Here's how the part is built. I have some questions about the finished solid (model axes, mm). Face numbers are marked on the shaded views. A direction names the side the tool comes from. Round coordinates to 2 decimals unless told otherwise and drop trailing zeros. Loops run counter-clockwise (first coordinate to the right, second up) from the corner with the lowest first, then second, coordinate; pieces in that order, holes last. Notation, with made-up numbers: M 16,84 L 34,84 A20 ccw 34,101 Z; hole C 17.5,-38 d1. An arc over 180 degrees is marked long. Write each question's results on one line, items separated by ' | '. Start each with the question number.
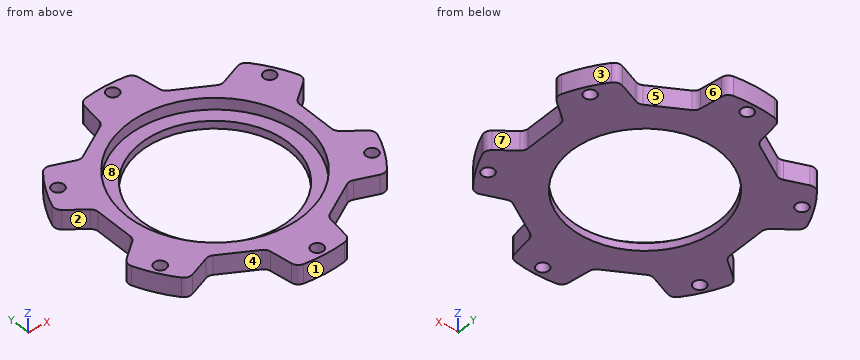
```python
from build123d import *

# Parameters (mm, degrees)
SKETCH_1_R          = 34
SKETCH_1_R_2        = 19
EXTRUDE_1_DEPTH     = 5
SKETCH_2_R          = 22.5
CUT_EXTRUDE_1_DEPTH = 3
SKETCH_3_R          = 1.55
CUT_EXTRUDE_2_DEPTH = 13
CUT_EXTRUDE_3_DEPTH = 13
FILLET_1_R          = 2


with BuildPart() as part:
    # 草图1 → 凸台-拉伸1 (new body)
    with BuildSketch(Plane.XY):
        Circle(SKETCH_1_R)
        Circle(SKETCH_1_R_2, mode=Mode.SUBTRACT)
    extrude(amount=EXTRUDE_1_DEPTH)

    # 草图2 → 切除-拉伸1 (cut)
    with BuildSketch(Plane.XY.offset(5)):
        Circle(SKETCH_2_R)
    extrude(amount=-CUT_EXTRUDE_1_DEPTH, mode=Mode.SUBTRACT)

    # 草图3 → 切除-拉伸2 (cut)
    with BuildSketch(Plane(origin=(0, 0, 0), x_dir=(-1, 0, 0), z_dir=(0, 0, -1))):
        with Locations((0, 31.5)):
            Circle(SKETCH_3_R)
        with Locations((27.279800219, 15.75)):
            Circle(SKETCH_3_R)
        with Locations((27.279800219, -15.75)):
            Circle(SKETCH_3_R)
        with Locations((0, -31.5)):
            Circle(SKETCH_3_R)
        with Locations((-27.279800219, -15.75)):
            Circle(SKETCH_3_R)
        with Locations((-27.279800219, 15.75)):
            Circle(SKETCH_3_R)
    extrude(amount=-CUT_EXTRUDE_2_DEPTH, mode=Mode.SUBTRACT)

    # 草图4 → 切除-拉伸3 (cut)
    with BuildSketch(Plane(origin=(0, 0, 0), x_dir=(-1, 0, 0), z_dir=(0, 0, -1))):
        with BuildLine():
            Line((-6.743785591, 33.324485831), (-7.903231695, 25.440443793))
            Line((-7.903231695, 25.440443793), (-18.080454761, 19.564621316))
            Line((-18.080454761, 19.564621316), (-25.487958502, 22.502532555))
            ThreePointArc((-25.487958502, 22.502532555), (-17, 29.444863729), (-6.743785591, 33.324485831))
        make_face()
        with BuildLine():
            Line((6.743785591, 33.324485831), (7.903231695, 25.440443793))
            Line((7.903231695, 25.440443793), (18.080454761, 19.564621316))
            Line((18.080454761, 19.564621316), (25.487958502, 22.502532555))
            ThreePointArc((25.487958502, 22.502532555), (17, 29.444863729), (6.743785591, 33.324485831))
        make_face()
        with BuildLine():
            Line((32.231744093, 10.821953276), (25.983686456, 5.875822477))
            Line((25.983686456, 5.875822477), (25.983686456, -5.875822477))
            Line((25.983686456, -5.875822477), (32.231744093, -10.821953276))
            ThreePointArc((32.231744093, -10.821953276), (34, 0), (32.231744093, 10.821953276))
        make_face()
        with BuildLine():
            Line((25.487958502, -22.502532555), (18.080454761, -19.564621316))
            Line((18.080454761, -19.564621316), (7.903231695, -25.440443793))
            Line((7.903231695, -25.440443793), (6.743785591, -33.324485831))
            ThreePointArc((6.743785591, -33.324485831), (17, -29.444863729), (25.487958502, -22.502532555))
        make_face()
        with BuildLine():
            Line((-6.743785591, -33.324485831), (-7.903231695, -25.440443793))
            Line((-7.903231695, -25.440443793), (-18.080454761, -19.564621316))
            Line((-18.080454761, -19.564621316), (-25.487958502, -22.502532555))
            ThreePointArc((-25.487958502, -22.502532555), (-17, -29.444863729), (-6.743785591, -33.324485831))
        make_face()
        with BuildLine():
            Line((-32.231744093, -10.821953276), (-25.983686456, -5.875822477))
            Line((-25.983686456, -5.875822477), (-25.983686456, 5.875822477))
            Line((-25.983686456, 5.875822477), (-32.231744093, 10.821953276))
            ThreePointArc((-32.231744093, 10.821953276), (-34, 0), (-32.231744093, -10.821953276))
        make_face()
    extrude(amount=-CUT_EXTRUDE_3_DEPTH, mode=Mode.SUBTRACT)

    # 圆角1
    fillet_1_edges = [part.edges().sort_by_distance(p)[0] for p in [
        (-25.983686456, -5.875822477, 2.5),
        (-25.983686456, 5.875822477, 2.5),
        (7.903231695, 25.440443793, 2.5),
        (18.080454761, 19.564621316, 2.5),
        (-18.080454761, 19.564621316, 2.5),
        (-7.903231695, 25.440443793, 2.5),
        (-6.743785591, 33.324485831, 2.5),
        (-25.487958502, 22.502532555, 2.5),
        (25.487958502, 22.502532555, 2.5),
        (6.743785591, 33.324485831, 2.5),
        (-32.231744093, 10.821953276, 2.5),
        (-32.231744093, -10.821953276, 2.5),
        (-25.487958502, -22.502532555, 2.5),
        (-6.743785591, -33.324485831, 2.5),
        (6.743785591, -33.324485831, 2.5),
        (25.487958502, -22.502532555, 2.5),
        (32.231744093, -10.821953276, 2.5),
        (32.231744093, 10.821953276, 2.5),
        (25.983686456, 5.875822477, 2.5),
        (25.983686456, -5.875822477, 2.5),
        (18.080454761, -19.564621316, 2.5),
        (7.903231695, -25.440443793, 2.5),
        (-7.903231695, -25.440443793, 2.5),
        (-18.080454761, -19.564621316, 2.5),
    ]]
    fillet(fillet_1_edges, radius=FILLET_1_R)


solid = part.part
```
Item 1: I'm going to push flat-ended pins straight in: pin 1 (1.5 mm diameter, centred on y = 1.5, z = 2, fed in from -X); pin 2 (3 mm diameter, centred on x = 11.5, z = 4, fed in from +Y); pin 3 (2 mm diameter, centred on y = 15.5, z = 2, fed in from -X); pin 4 (1.9 mm diameter, centred on x = -27.28, y = 15.75, fed in from +Z). Where does each tip first touch, or does it pass through?
Item 2: I need wall thicknesses on L1, parallel to Y at x = 0, z = 1.5; L2, parallel to Y at x = 0, z = 3.9; L3, parallel to X at y = 0, z = 1.15. Which ranges of each line are inside material? Lowest first, please.
Item 3: If we section it at C-C on z = 0.75: Count the separate pieces of the cut face and the enclosed holes in it, and give its area (3 significant figures).
Item 4: If we section it at B-B on y = 0: Please give me the cut outline in (x, z).
Item 5: If we mould it in two halves opening along Y, with no side actions, what happens to the marked faces 1, 2 and 3? For each: released by +Y, released by -Y, zero draft, split by the parting line, or undercut.
Item 6: If we section it at D-D on x = -12: Please give me the cut outline in (y, z).
Item 7: If we section it at A-A on x = 0: Please give me the cut outline in (y, z).
Item 8: Which directions (+Z, -Z, +X, -X, +Y, -Y) give clear straight access to the entire face, cutting with the end or side of a thin tool? Please do the marked faces 4, 5, 6, 7 and 8.
Numbers:
1) pin 1: x = -25.98 | pin 2: y = 24.23 | pin 3: x = -30.75 | pin 4: through
2) L1: -34 to -33.05, -29.95 to -19, 19 to 29.95, 33.05 to 34 | L2: -34 to -33.05, -29.95 to -22.5, 22.5 to 29.95, 33.05 to 34 | L3: -25.98 to -19, 19 to 25.98
3) separate pieces: 1 | enclosed holes: 7 | area: 1,670 mm²
4) outline: M -25.98,0 L -19,0 L -19,2 L -22.5,2 L -22.5,5 L -25.98,5 Z; M 19,0 L 25.98,0 L 25.98,5 L 22.5,5 L 22.5,2 L 19,2 Z
5) face 1: released by -Y | face 2: undercut | face 3: released by +Y
6) outline: M -23.08,0 L -14.73,0 L -14.73,2 L -19.03,2 L -19.03,5 L -23.08,5 Z; M 14.73,0 L 23.08,0 L 23.08,5 L 19.03,5 L 19.03,2 L 14.73,2 Z
7) outline: M -34,0 L -33.05,0 L -33.05,5 L -34,5 Z; M -29.95,0 L -19,0 L -19,2 L -22.5,2 L -22.5,5 L -29.95,5 Z; M 19,0 L 29.95,0 L 29.95,5 L 22.5,5 L 22.5,2 L 19,2 Z; M 33.05,0 L 34,0 L 34,5 L 33.05,5 Z
8) face 4: +Z, -Z, -Y | face 5: +Z, -Z, +Y | face 6: +Z, -Z, +X, +Y | face 7: +Z, -Z, +X | face 8: +Z
